CAD build for the part. Positions are in the model's coordinates, mm. A direction names the side the tool comes from. Give positions to 0.01 mm unless a question says otherwise; leave off trailing zeros. Write each loop counter-clockwise with the first axis right and the second up, starting at its lowest first coordinate (ties: lowest second). Pieces come first, ordered by that corner, then holes. Notation, with made-up numbers: (29, -28.75) -> (51, -28.75) arc R38 cw to (51, 10.25) -> close; hole circle Ø4 at (79, 45.25). An arc over 180 degrees is marked (long way). Answer as a JSON object with one key per item and string values.
```python
from build123d import *

# Parameters (mm, degrees)
F0_R     = 20
F1_DEPTH = 3


with BuildPart() as f1:
    # F0 (on Front) → F1 (new body)
    with BuildSketch(Plane.XZ):
        with BuildLine():
            ThreePointArc((-39.2839784876, -3.7990042795), (-32.8873709815, -1.9913052768), (-27.4364980034, 1.8129485328))
            Line((-27.4364980034, 1.8129485328), (-27.9683212743, 2.7340934586))
            Line((-27.9683212743, 2.7340934586), (-39.2839784876, -3.7990042795))
        make_face()
        with BuildLine():
            Line((-2.9683212743, -40.5671767306), (-3.5001445452, -39.6460318047))
            ThreePointArc((-3.5001445452, -39.6460318047), (-9.5201614758, -42.4644993718), (-14.2839784876, -47.1002744687))
            Line((-14.2839784876, -47.1002744687), (-2.9683212743, -40.5671767306))
        make_face()
        with BuildLine():
            Line((-16.4490833879, -17.2178118252), (-27.4364980034, 1.8129485328))
            ThreePointArc((-27.4364980034, 1.8129485328), (-32.8873709815, -1.9913052768), (-39.2839784876, -3.7990042795))
            Line((-39.2839784876, -3.7990042795), (-41.4490833879, -5.0490281765))
            Line((-41.4490833879, -5.0490281765), (-16.4490833879, -19.4827849062))
            Line((-16.4490833879, -19.4827849062), (-16.4490833879, -17.2178118252))
        make_face()
        with BuildLine():
            Line((-16.4490833879, -50.8503461597), (-16.4490833879, -48.3502983657))
            Line((-16.4490833879, -48.3502983657), (-41.4490833879, -62.7840550955))
            Line((-41.4490833879, -62.7840550955), (-39.4875591608, -63.916541636))
            Line((-39.4875591608, -63.916541636), (-17.5127299297, -63.916541636))
            ThreePointArc((-17.5127299297, -63.916541636), (-18.0818738821, -57.2938202594), (-16.4490833879, -50.8503461597))
        make_face()
        with BuildLine():
            Line((-14.2839784876, -47.1002744687), (-16.4490833879, -48.3502983657))
            Line((-16.4490833879, -48.3502983657), (-16.4490833879, -50.8503461597))
            ThreePointArc((-16.4490833879, -50.8503461597), (-15.4683212743, -48.916541636), (-14.2839784876, -47.1002744687))
        make_face()
        with BuildLine():
            Line((-14.4875591608, -20.6152714468), (-16.4490833879, -19.4827849062))
            Line((-16.4490833879, -19.4827849062), (-16.4490833879, -48.3502983657))
            Line((-16.4490833879, -48.3502983657), (-14.2839784876, -47.1002744687))
            ThreePointArc((-14.2839784876, -47.1002744687), (-9.5201614758, -42.4644993718), (-3.5001445452, -39.6460318047))
            Line((-3.5001445452, -39.6460318047), (-14.4875591608, -20.6152714468))
        make_face()
        with BuildLine():
            Line((-16.4490833879, -63.916541636), (-16.4490833879, -50.8503461597))
            ThreePointArc((-16.4490833879, -50.8503461597), (-18.0818738821, -57.2938202594), (-17.5127299297, -63.916541636))
            Line((-17.5127299297, -63.916541636), (-16.4490833879, -63.916541636))
        make_face()
        Polygon((-14.4875591608, -20.6152714468), (-16.4490833879, -17.2178118252), (-16.4490833879, -19.4827849062), align=None)
        with BuildLine():
            ThreePointArc((-55.4616687723, 1.8129485328), (-49.186921985, 34.5259596544), (-21.4490833879, 16.083458364))
            ThreePointArc((-21.4490833879, 16.083458364), (-23.0065820975, 8.3456197669), (-27.4364980034, 1.8129485328))
            Line((-27.4364980034, 1.8129485328), (-16.4490833879, -17.2178118252))
            Line((-16.4490833879, -17.2178118252), (-16.4490833879, 46.083458364))
            Line((-16.4490833879, 46.083458364), (-66.4490833879, 46.083458364))
            Line((-66.4490833879, 46.083458364), (-66.4490833879, -17.2178118252))
            Line((-66.4490833879, -17.2178118252), (-55.4616687723, 1.8129485328))
        make_face()
        with BuildLine():
            Line((-79.3980222305, -39.6460318047), (-68.4106076149, -20.6152714468))
            Line((-68.4106076149, -20.6152714468), (-123.2311156906, -52.2659065414))
            Line((-123.2311156906, -52.2659065414), (-98.2311156906, -95.5671767306))
            Line((-98.2311156906, -95.5671767306), (-43.4106076149, -63.916541636))
            Line((-43.4106076149, -63.916541636), (-65.385436846, -63.916541636))
            ThreePointArc((-65.385436846, -63.916541636), (-102.0708616528, -68.916541636), (-79.3980222305, -39.6460318047))
        make_face()
        with BuildLine():
            Line((40.3329489149, -52.2659065414), (-14.4875591608, -20.6152714468))
            Line((-14.4875591608, -20.6152714468), (-3.5001445452, -39.6460318047))
            ThreePointArc((-3.5001445452, -39.6460318047), (13.9549421296, -42.9941261953), (21.8521868014, -58.916541636))
            ThreePointArc((21.8521868014, -58.916541636), (4.372272651, -78.7571355613), (-17.5127299297, -63.916541636))
            Line((-17.5127299297, -63.916541636), (-39.4875591608, -63.916541636))
            Line((-39.4875591608, -63.916541636), (15.3329489149, -95.5671767306))
            Line((15.3329489149, -95.5671767306), (40.3329489149, -52.2659065414))
        make_face()
        with BuildLine():
            Line((-41.4490833879, -62.7840550955), (-66.4490833879, -48.3502983657))
            Line((-66.4490833879, -48.3502983657), (-66.4490833879, -50.8503461597))
            ThreePointArc((-66.4490833879, -50.8503461597), (-65.1796432708, -54.7949766289), (-64.7503535771, -58.916541636))
            ThreePointArc((-64.7503535771, -58.916541636), (-64.9097596517, -61.4366274856), (-65.385436846, -63.916541636))
            Line((-65.385436846, -63.916541636), (-43.4106076149, -63.916541636))
            Line((-43.4106076149, -63.916541636), (-41.4490833879, -62.7840550955))
        make_face()
        with BuildLine():
            Line((-66.4490833879, -48.3502983657), (-66.4490833879, -19.4827849062))
            Line((-66.4490833879, -19.4827849062), (-68.4106076149, -20.6152714468))
            Line((-68.4106076149, -20.6152714468), (-79.3980222305, -39.6460318047))
            ThreePointArc((-79.3980222305, -39.6460318047), (-73.3780052999, -42.4644993718), (-68.6141882881, -47.1002744687))
            Line((-68.6141882881, -47.1002744687), (-66.4490833879, -48.3502983657))
        make_face()
        with BuildLine():
            ThreePointArc((-43.6141882881, -3.7990042795), (-50.0107957942, -1.9913052768), (-55.4616687723, 1.8129485328))
            Line((-55.4616687723, 1.8129485328), (-66.4490833879, -17.2178118252))
            Line((-66.4490833879, -17.2178118252), (-66.4490833879, -19.4827849062))
            Line((-66.4490833879, -19.4827849062), (-41.4490833879, -5.0490281765))
            Line((-41.4490833879, -5.0490281765), (-43.6141882881, -3.7990042795))
        make_face()
        Polygon((-16.4490833879, -19.4827849062), (-41.4490833879, -5.0490281765), (-66.4490833879, -19.4827849062), (-66.4490833879, -48.3502983657), (-41.4490833879, -62.7840550955), (-16.4490833879, -48.3502983657), align=None)
        with Locations((-41.4490833879, -33.916541636)):
            Circle(F0_R, mode=Mode.SUBTRACT)
        with BuildLine():
            ThreePointArc((-64.7503535771, -58.916541636), (-65.1796432708, -54.7949766289), (-66.4490833879, -50.8503461597))
            Line((-66.4490833879, -50.8503461597), (-66.4490833879, -63.916541636))
            Line((-66.4490833879, -63.916541636), (-65.385436846, -63.916541636))
            ThreePointArc((-65.385436846, -63.916541636), (-64.9097596517, -61.4366274856), (-64.7503535771, -58.916541636))
        make_face()
        Polygon((-39.4875591608, -63.916541636), (-41.4490833879, -62.7840550955), (-43.4106076149, -63.916541636), align=None)
        Polygon((-66.4490833879, -19.4827849062), (-66.4490833879, -17.2178118252), (-68.4106076149, -20.6152714468), align=None)
        with BuildLine():
            ThreePointArc((-68.6141882881, -47.1002744687), (-73.3780052999, -42.4644993718), (-79.3980222305, -39.6460318047))
            Line((-79.3980222305, -39.6460318047), (-79.9298455014, -40.5671767306))
            Line((-79.9298455014, -40.5671767306), (-68.6141882881, -47.1002744687))
        make_face()
        with BuildLine():
            ThreePointArc((-39.2839784876, -3.7990042795), (-41.4490833879, -3.916541636), (-43.6141882881, -3.7990042795))
            Line((-43.6141882881, -3.7990042795), (-41.4490833879, -5.0490281765))
            Line((-41.4490833879, -5.0490281765), (-39.2839784876, -3.7990042795))
        make_face()
        with BuildLine():
            Line((-66.4490833879, -50.8503461597), (-66.4490833879, -48.3502983657))
            Line((-66.4490833879, -48.3502983657), (-68.6141882881, -47.1002744687))
            ThreePointArc((-68.6141882881, -47.1002744687), (-67.4298455014, -48.916541636), (-66.4490833879, -50.8503461597))
        make_face()
        with BuildLine():
            Line((-54.9298455014, 2.7340934586), (-55.4616687723, 1.8129485328))
            ThreePointArc((-55.4616687723, 1.8129485328), (-50.0107957942, -1.9913052768), (-43.6141882881, -3.7990042795))
            Line((-43.6141882881, -3.7990042795), (-54.9298455014, 2.7340934586))
        make_face()
    extrude(amount=F1_DEPTH)


solid = f1.part
```
1) Slice it at D-D (x = -32.5). List the corners of the cut face in (y, z), then the cut area to 3 significant figures.
Model answer:
{"outline": "(-3, -67.95) -> (0, -67.95) -> (0, -51.8) -> (-3, -51.8) -> close; (-3, -16.03) -> (0, -16.03) -> (0, 0.12) -> (-3, 0.12) -> close; (-3, 33.97) -> (0, 33.97) -> (0, 46.08) -> (-3, 46.08) -> close", "area": "133 mm2"}
2) Mould opens along Z. For faces 4 (the flat face through (-8.71, -1.48, -43.88)), 5 (the flat face through (27.66, -1.48, -74.22)), 6 (the flat face through (13.306, -1.479, -36.662)) say: released by +Z, released by -Z, zero draft, split by the parting line, or undercut.
Model answer:
{"face 4": "undercut", "face 5": "released by -Z", "face 6": "released by +Z"}
3) Slice it at C-C (y = -1.15). State how many separate pieces and enclosed holes the cut face has, then the cut area to 3 significant figures.
Model answer:
{"separate pieces": "1", "enclosed holes": "4", "area": "6,000 mm2"}
4) Wall check: probe 1 along Z at (x, y) = (-56, -1.4); probe 2 along Z at (x, y) = (-48, -0.05); probe 3 along X at (y, z) = (-2.8, 39.5). Give the ranges that are in metal, low to high.
Model answer:
{"probe 1": "z = -71.19 to -47.64, -20.2 to 2.36, 29.8 to 46.08", "probe 2": "z = -66.57 to -52.81, -15.02 to -1.27, 34.98 to 46.08", "probe 3": "x = -66.45 to -16.45"}
5) Slice it at A-A (x = 8). List the corners of the cut face in (y, z).
Model answer:
{"outline": "(-3, -91.33) -> (0, -91.33) -> (0, -77.95) -> (-3, -77.95) -> close; (-3, -39.88) -> (0, -39.88) -> (0, -33.6) -> (-3, -33.6) -> close"}
6) 3-axis set-ups, long thin cutter, end or side, ignore diameter. For faces 1 (the flat face through (-74.35, -1.48, -43.79)), 2 (the flat face through (-71.2, -1.48, -79.96)), 3 (the flat face through (-95.44, -1.48, -36.22)): which of +Z, -Z, +X, -X, +Y, -Y reach the whole face in a straight line?
Model answer:
{"face 1": "+Y, -Y", "face 2": "-Z, +Y, -Y", "face 3": "+Z, -X, +Y, -Y"}
7) Pin check, flat tips, straight feed: pin 1 (0.9 mm diameter, centred on x = -42, y = -1, fed in from -Z); pin 2 (0.9 mm diameter, centred on y = -1, z = 2, fed in from -X); pin 3 (0.9 mm diameter, centred on y = -1.5, z = -56, fed in from -X); pin 4 (24 mm diameter, centred on x = -41.45, z = -33.92, fed in from +Y). Stop position of each tip, or through.
Model answer:
{"pin 1": "stops at z = -63.92", "pin 2": "stops at x = -66.45", "pin 3": "stops at x = -121.34", "pin 4": "passes through"}
8) Slice it at B-B (z = 14). List the corners of the cut face in (x, y).
Model answer:
{"outline": "(-66.45, -3) -> (-61.34, -3) -> (-61.34, 0) -> (-66.45, 0) -> close; (-21.56, -3) -> (-16.45, -3) -> (-16.45, 0) -> (-21.56, 0) -> close"}
